Here's the drawing with two shaded views (mm, measured from the low corner). I have some questions. A direction names the side the tool comes from. Round coordinates to 2 decimals unless told otherwise and drop trailing zeros. Loops run counter-clockwise (first coordinate to the right, second up) from the corner with the lowest first, then second, coordinate; pieces in that order, holes last.
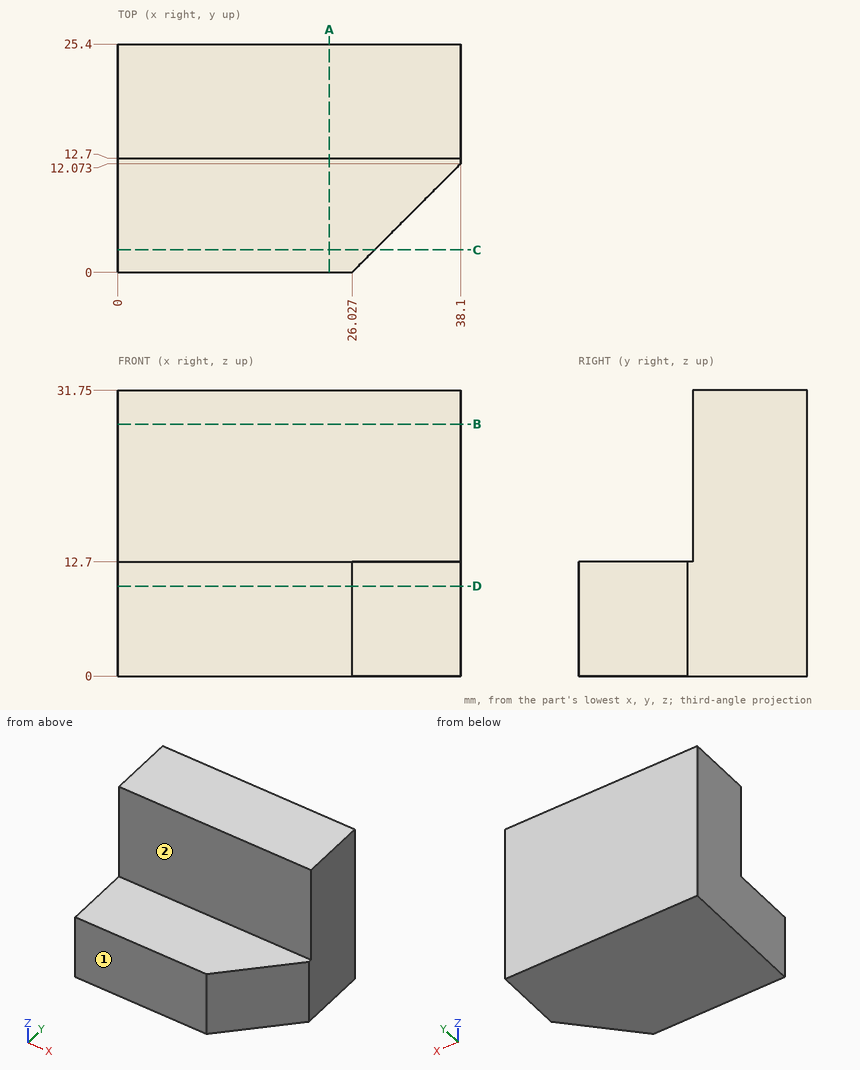
Item 1: For the marked faces 1 and 2, which set-ups out of +Z, -Z, +X, -X, +Y, -Y let a thin tool reach every point of the face, with its end or its side?
Results list:
face 1: +Z, -Z, +X, -X, -Y
face 2: +Z, +X, -X, -Y
Item 2: If we section it at A-A, the plane x = 23.5: Please give me the cut outline in (y, z).
Results list:
outline: (0, 0) - (25.4, 0) - (25.4, 31.75) - (12.7, 31.75) - (12.7, 12.7) - (0, 12.7) - close
Item 3: If I drill on line 1 along Y through (x, z) = (35, 13); line 2 along Z through (x, y) = (5, 6); line 3 along Y through (x, z) = (32.5, 11), over which ranges is the centre line in solid material (lowest first)?
Results list:
line 1: y = 12.7 to 25.4
line 2: z = 0 to 12.7
line 3: y = 6.47 to 25.4
Item 4: Will these pins go through, and if not, where does the flat tip stop? pin 1 (5.5 mm diameter, centred on x = 18, z = 22.5, fed in from -Y); pin 2 (1.5 mm diameter, centred on y = 11, z = 19.5, fed in from -X).
Results list:
pin 1: stops at y = 12.7
pin 2: passes through
Item 5: If we section it at B-B, the plane z = 28: Please give me the cut outline in (x, y), then the cut area to 3 significant figures.
Results list:
outline: (0, 12.7) - (38.1, 12.7) - (38.1, 25.4) - (0, 25.4) - close
area: 484 mm2
Item 6: If we section it at C-C, the plane y = 2.5: Please give me the cut outline in (x, z).
Results list:
outline: (0, 0) - (28.53, 0) - (28.53, 12.7) - (0, 12.7) - close
Item 7: If we section it at D-D, the plane z = 10: Please give me the cut outline in (x, y), then the cut area to 3 significant figures.
Results list:
outline: (0, 0) - (26.03, 0) - (38.1, 12.07) - (38.1, 25.4) - (0, 25.4) - close
area: 895 mm2
